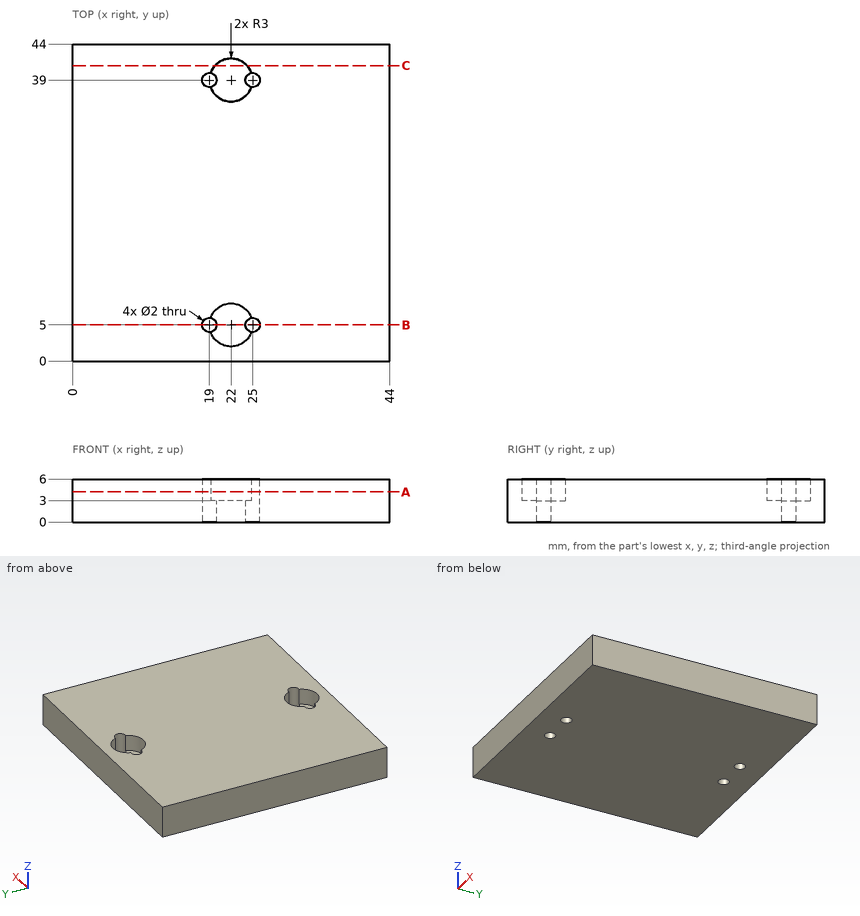
Here's the drawing with two shaded views (mm, measured from the low corner). I have some questions. Give positions to 0.01 mm unless a question says otherwise; leave off trailing zeros. Loops run counter-clockwise (first coordinate to the right, second up) from the corner with the lowest first, then second, coordinate; pieces in that order, holes last. Notation, with made-up numbers: (83.5, -27.75) -> (96.5, -27.75) arc R12 cw to (96.5, -14.75) -> close; hole circle Ø10 at (-20, 21.25). An arc over 180 degrees is marked (long way). Use one line per item in the form item = value.
1) If we section it at A-A (z = 4.2): Please give me the cut outline in (x, y).
Answers:
outline = (0, 0) -> (44, 0) -> (44, 44) -> (0, 44) -> close; hole (19.17, 4.01) arc R3 ccw to (24.83, 4.01) arc R1 ccw (long way) to (24.83, 5.99) arc R3 ccw to (19.17, 5.99) arc R1 ccw (long way) to start; hole (19.17, 38.01) arc R3 ccw to (24.83, 38.01) arc R1 ccw (long way) to (24.83, 39.99) arc R3 ccw to (19.17, 39.99) arc R1 ccw (long way) to start
2) If we section it at C-C (y = 41): Please give me the cut outline in (x, z), plus the area to 3 significant figures.
Answers:
outline = (0, 0) -> (44, 0) -> (44, 6) -> (24.24, 6) -> (24.24, 3) -> (19.76, 3) -> (19.76, 6) -> (0, 6) -> close
area = 251 mm²
3) I need wall thicknesses on line 1 along Y through (x, z) = (25, 1.45); line 2 along X through (y, z) = (39, 2.05); line 3 along X through (y, z) = (4.5, 3.6). Which ranges of each line are inside material? Lowest first, please.
Answers:
line_1 = 0 to 4, 6 to 38, 40 to 44
line_2 = 0 to 18, 20 to 24, 26 to 44
line_3 = 0 to 18.13, 25.87 to 44
4) If we section it at B-B (y = 5): Please give me the cut outline in (x, z), plus the area to 3 significant figures.
Answers:
outline = (0, 0) -> (18, 0) -> (18, 6) -> (0, 6) -> close; (20, 0) -> (24, 0) -> (24, 3) -> (20, 3) -> close; (26, 0) -> (44, 0) -> (44, 6) -> (26, 6) -> close
area = 228 mm²
